For this review, take the finished solid that the model builds, in its own axes (mm). A direction names the side the tool comes from. Give positions to 0.01 mm unless a question says otherwise; leave off trailing zeros. Loops run counter-clockwise (first coordinate to the right, second up) from the corner with the lowest first, then second, coordinate; pieces in that order, holes last. Notation, with made-up numbers: (7.25, -4.75) -> (17.25, -4.75) arc R25 ccw to (17.25, 15.25) -> close; hole circle Ø9 at (55, 53.25). An arc over 180 degrees is marked (long way). One line per question, with ' | ' between items. Start each with the question number.
(1) Wall thickness on probe 1 along Y at (x, z) = (-40, 0.2); probe 2 along Y at (x, z) = (17, 0.5) (3 decimals); probe 3 along X at (y, z) = (37, 1.75): over which ranges is each line inside the solid? List them lowest first.
(2) Consider section B-B (x = -38). Write out the cut boundary in (y, z), and give its area (3 significant figures).
(3) Consider section C-C (y = 33). Write out the cut boundary in (x, z).
(4) Consider section A-A (y = 0). Write out the cut boundary in (x, z) (3 decimals), and give its area (3 significant figures).
(5) Consider section D-D (x = -9). Write out the cut boundary in (y, z), and give its area (3 significant figures).
(6) Insertion check: P1, Ø1, axis at y = -14, z = 1, coming from the +X side; P2, Ø8, axis at x = 19.5, y = 13, coming from the +Z side; P3, Ø0.6, axis at y = 20, z = 1.5, coming from the +X side; P4, Ø4, axis at x = -17.46, y = 34.92, coming from the -Z side. Each pin has a flat end and moves straight along its axis. Give the tip position at first contact, or say it passes through.
(7) Tool access review of faces 1 (the flat face through (17, -16, 2.032)), 2 (the flat face through (11.323, 13.049, 1.002)): name each direction out of +Z, -Z, +X, -X, +Y, -Y from which nothing blocks a thin tool from reaching the whole face with its end or side.
from build123d import *

# Parameters (mm, degrees)
F0_R     = 52.3875
F1_DEPTH = 2.54
F2_R     = 2.54
F3_W     = 63.5
F3_H     = 50.8
F4_DEPTH = 0.508
F5_R     = 52.3875
F5_R_2   = 46.99
F5_R_3   = 2.38125
F5_R_4   = 3.175
F6_DEPTH = 25.4
F7_W     = 1.524
F7_H     = 15.875
F8_DEPTH = 25.4


# Not quite as in the source:
# - a feature names something its author has since deleted; it is built from what else it names


with BuildPart() as f1:
    # F0 (on Top) → F1 (new body)
    with BuildSketch(Plane.XY):
        Circle(F0_R)
        Polygon((-34.925, 25.4), (-33.3375, 25.4), (-30.1625, 25.4), (-19.05, 25.4), (-19.05, 15.24), (-21.844, 10.795), (-19.05, 9.525), (-17.4625, 9.525), (-14.2875, 9.525), (-11.4935, 10.795), (-14.2875, 15.24), (-14.2875, 25.4), (-3.175, 25.4), (-3.175, 15.24), (-5.969, 10.795), (-3.175, 9.525), (-1.5875, 9.525), (1.5875, 9.525), (4.3815, 10.795), (1.5875, 15.24), (1.5875, 25.4), (12.7, 25.4), (12.7, 15.24), (9.906, 10.795), (12.7, 9.525), (14.2875, 9.525), (17.4625, 9.525), (20.2565, 10.795), (17.4625, 15.24), (17.4625, 25.4), (28.575, 25.4), (28.575, -25.4), (17.4625, -25.4), (17.4625, -15.24), (20.2565, -10.795), (17.4625, -9.525), (14.2875, -9.525), (12.7, -9.525), (9.906, -10.795), (12.7, -15.24), (12.7, -25.4), (1.5875, -25.4), (1.5875, -15.24), (4.3815, -10.795), (1.5875, -9.525), (-1.5875, -9.525), (-3.175, -9.525), (-5.969, -10.795), (-3.175, -15.24), (-3.175, -25.4), (-14.2875, -25.4), (-14.2875, -15.24), (-11.4935, -10.795), (-14.2875, -9.525), (-17.4625, -9.525), (-19.05, -9.525), (-21.844, -10.795), (-19.05, -15.24), (-19.05, -25.4), (-30.1625, -25.4), (-33.3375, -25.4), (-34.925, -25.4), align=None, mode=Mode.SUBTRACT)
        Polygon((-33.3375, 9.525), (-30.1625, 9.525), (-27.3685, 10.795), (-30.1625, 15.24), (-30.1625, 25.4), (-33.3375, 25.4), align=None)
        Polygon((-33.3375, -9.525), (-33.3375, -25.4), (-30.1625, -25.4), (-30.1625, -15.24), (-27.3685, -10.795), (-30.1625, -9.525), align=None)
    extrude(amount=F1_DEPTH)

    # F2
    f2_edges = [f1.edges().sort_by_distance(p)[0] for p in [
        (-30.1625, 25.4, 1.27),
        (-14.2875, 25.4, 1.27),
        (1.5875, 25.4, 1.27),
        (17.4625, 25.4, 1.27),
        (17.4625, -25.4, 1.27),
        (1.5875, -25.4, 1.27),
        (-14.2875, -25.4, 1.27),
        (-30.1625, -25.4, 1.27),
        (-19.05, -25.4, 1.27),
        (-3.175, -25.4, 1.27),
        (12.7, -25.4, 1.27),
        (12.7, 25.4, 1.27),
        (-3.175, 25.4, 1.27),
        (-19.05, 25.4, 1.27),
    ]]
    fillet(f2_edges, radius=F2_R)

    # F3 (on face) → F4 (cut)
    with BuildSketch(Plane.XY.offset(2.54)):
        with Locations((-3.175, 0)):
            Rectangle(F3_W, F3_H)
    extrude(amount=-F4_DEPTH, mode=Mode.SUBTRACT)

    # F5 (on face) → F6 (cut)
    with BuildSketch(Plane.XY.offset(2.54)):
        Circle(F5_R)
        Circle(F5_R_2, mode=Mode.SUBTRACT)
        with Locations((-38.4948291982, 22.225)):
            Circle(F5_R_3)
        with Locations((-38.4948291982, -22.225)):
            Circle(F5_R_3)
        with Locations((38.4948291982, -22.225)):
            Circle(F5_R_3)
        with Locations((38.4948291982, 22.225)):
            Circle(F5_R_3)
        with Locations((17.4625, -34.925)):
            Circle(F5_R_4)
        with Locations((17.4625, 34.925)):
            Circle(F5_R_4)
        with Locations((-17.4625, 34.925)):
            Circle(F5_R_4)
        with Locations((-17.4625, -34.925)):
            Circle(F5_R_4)
    extrude(amount=-F6_DEPTH, mode=Mode.SUBTRACT)

    # F7 (on face) → F8 (cut)
    with BuildSketch(Plane.XY.offset(2.54)):
        with Locations((-16.66875, 17.4625)):
            Rectangle(F7_W, F7_H)
        with Locations((-0.79375, 17.4625)):
            Rectangle(F7_W, F7_H)
        with Locations((15.08125, 17.4625)):
            Rectangle(F7_W, F7_H)
        with Locations((-16.66875, -17.4625)):
            Rectangle(F7_W, F7_H)
        with Locations((-0.79375, -17.4625)):
            Rectangle(F7_W, F7_H)
        with Locations((15.08125, -17.4625)):
            Rectangle(F7_W, F7_H)
    extrude(amount=-F8_DEPTH, mode=Mode.SUBTRACT)


solid = f1.part
A:
1) probe 1: y = -24.66 to -24.07, -20.38 to 20.38, 24.07 to 24.66 | probe 2: y = -43.807 to -38.066, -31.784 to -9.525, 9.525 to 31.784, 38.066 to 43.807 | probe 3: x = -28.97 to -19.87, -15.06 to 15.06, 19.87 to 28.97
2) outline: (-27.64, 0) -> (-24.55, 0) -> (-24.55, 2.54) -> (-27.64, 2.54) -> close; (-19.9, 0) -> (19.9, 0) -> (19.9, 2.54) -> (-19.9, 2.54) -> close; (24.55, 0) -> (27.64, 0) -> (27.64, 2.54) -> (24.55, 2.54) -> close | area: 117 mm^2
3) outline: (-33.45, 0) -> (-19.99, 0) -> (-19.99, 2.54) -> (-33.45, 2.54) -> close; (-14.94, 0) -> (14.94, 0) -> (14.94, 2.54) -> (-14.94, 2.54) -> close; (19.99, 0) -> (33.45, 0) -> (33.45, 2.54) -> (19.99, 2.54) -> close
4) outline: (-46.99, 0) -> (-34.925, 0) -> (-34.925, 2.54) -> (-46.99, 2.54) -> close; (28.575, 0) -> (46.99, 0) -> (46.99, 2.54) -> (28.575, 2.54) -> close | area: 77.4 mm^2
5) outline: (-46.12, 0) -> (-25.4, 0) -> (-25.4, 2.54) -> (-46.12, 2.54) -> close; (25.4, 0) -> (46.12, 0) -> (46.12, 2.54) -> (25.4, 2.54) -> close | area: 105 mm^2
6) P1: stops at x = 45.01 | P2: stops at z = 2.03 | P3: stops at x = 42.66 | P4: passes through
7) face 1: +Z | face 2: +Z, -Z
